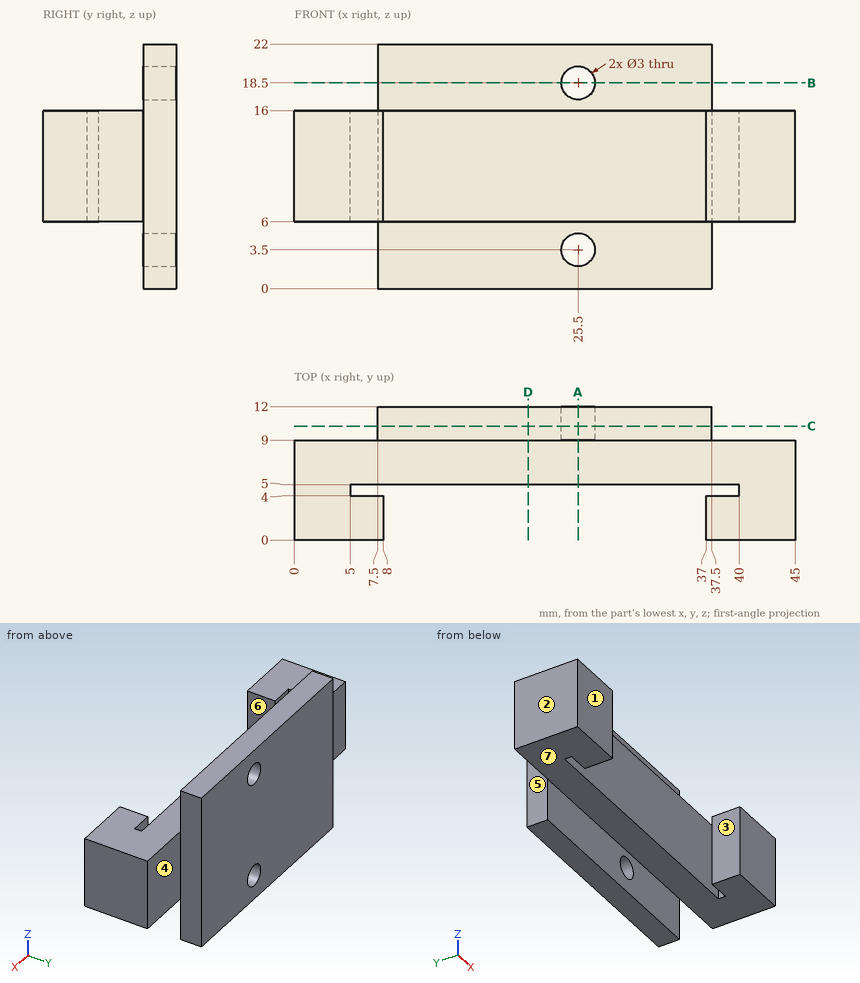
For this review, use the dimensioned drawing (mm, ordinates from the lowest corner) and the shaded views. A direction names the side the tool comes from. Coordinates: 2 decimals unless noted, no trailing zeros. Order: outer loops, then holes, each group sorted by start corner. A loop starts at its lowest first (then second) coordinate and runs counter-clockwise, first axis right, second up. Notation, with made-up numbers: M 82,24 L 97,24 A28 ccw 97,48 Z; hole C 33,-3 d3. An arc over 180 degrees is marked long. Answer as a JSON object with one key per item and string values. Group by question number.
1) Add section B-B, the plane z = 18.5. Write out the cut boundary in (x, y), then the cut area to 3 significant figures.
2) Add section D-D, the plane x = 21. Write out the cut boundary in (y, z).
3) Wall thickness on L1, parallel to Z at x = 25.5, y = 10.1; L2, parallel to X at y = 4.5, z = 8.5; L3, parallel to X at y = 10.5, z = 18.5: over which ranges is each line inside the solid? List them lowest first.
4) Add section C-C, the plane y = 10.25. Write out the cut boundary in (x, z).
5) Tool access review of the marked faces 4, 5, 6 and 7: name each direction out of +Z, -Z, +X, -X, +Y, -Y from which nothing blocks a thin tool from reaching the whole face with its end or side.
6) Mouldability with a two-part tool opening along X and no side actions: class the marked faces 1, 2 and 3 as pulls with the +X half, pulls with the -X half, needs draft (parallel to the pull), parting line crosses it, or undercut.
7) For pin 1 (0.9 mm diameter, centred on y = 11, z = 7.5, fed in from -X); pin 2 (2.5 mm diameter, centred on y = 10, z = 14, fed in from +X); pin 3 (1.5 mm diameter, centred on x = 6.5, z = 9.5, fed in from +Y); pin 4 (6 mm diameter, centred on x = 15, z = 5, fed in from -Y), all flat-tipped, find the tip position at first contact; note any pin that passes through.
8) Add section A-A, the plane x = 25.5. Write out the cut boundary in (y, z).
Computed values:
{
 "1": {"outline": "M 7.5,9 L 24,9 L 24,12 L 7.5,12 Z; M 27,9 L 37.5,9 L 37.5,12 L 27,12 Z", "area": "81.0 mm^2"},
 "2": {"outline": "M 5,6 L 9,6 L 9,0 L 12,0 L 12,22 L 9,22 L 9,16 L 5,16 Z"},
 "3": {"L1": "z = 0 to 2, 5 to 17, 20 to 22", "L2": "x = 0 to 5, 40 to 45", "L3": "x = 7.5 to 24, 27 to 37.5"},
 "4": {"outline": "M 7.5,0 L 37.5,0 L 37.5,22 L 7.5,22 Z; hole C 25.5,3.5 d3; hole C 25.5,18.5 d3"},
 "5": {"face 4": "+Z, -Z, +X, +Y", "face 5": "+Z, -Z, -X, +Y", "face 6": "+Z, -Z, -Y", "face 7": "-Z, +X, -X, -Y"},
 "6": {"face 1": "needs draft", "face 2": "pulls with the -X half", "face 3": "undercut"},
 "7": {"pin 1": "stops at x = 7.5", "pin 2": "stops at x = 45", "pin 3": "stops at y = 9", "pin 4": "stops at y = 5"},
 "8": {"outline": "M 5,6 L 9,6 L 9,5 L 12,5 L 12,17 L 9,17 L 9,16 L 5,16 Z; M 9,0 L 12,0 L 12,2 L 9,2 Z; M 9,20 L 12,20 L 12,22 L 9,22 Z"}
}
